CAD build for the part. Positions are in the model's coordinates, mm. Give positions to 0.01 mm unless a question says otherwise; leave off trailing zeros. Order: outer loops, then holes, each group sorted by start corner. A loop starts at its lowest first (then second) coordinate and runs counter-clockwise, first axis right, second up.
Item 1: Flat gauge pins, fed straight in: P1, Ø1, axis at x = 28, y = 3, coming from the +Z side; P2, Ø2, axis at x = 19.5, z = 1, coming from the -Y side. Where does each tip first touch, or does it go through?
Item 2: Band-saw the part on A-A on x = 25. Give the cut face in (y, z).
Item 3: Band-saw the part on B-B on x = 32. Give the cut face in (y, z).
Item 4: Wall check: L1, parallel to X at y = 1.8, z = -1.5 (3 decimals); L2, parallel to Y at x = 32, z = 0.65; L3, parallel to Y at x = 33, z = 0.3. Give the ranges that are in metal, low to high.
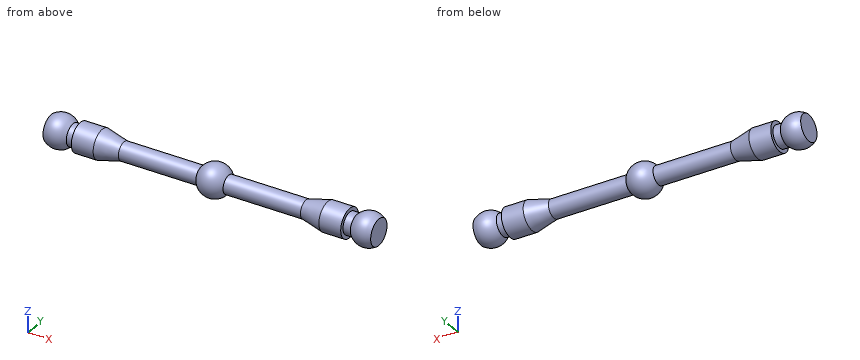
Autodesk Inventor part; units mm, degrees
ref_plane "YZ Plane" through (0, 0, 0) normal (1, 0, 0) x (0, 1, 0)
ref_plane "XZ Plane" through (0, 0, 0) normal (0, 1, 0) x (-1, 0, 0)
ref_plane "XY Plane" through (0, 0, 0) normal (0, 0, 1) x (1, 0, 0)
sketch "Sketch1" plane through (0, 0, 0) normal (0, 0, 1) x (1, 0, 0)
  line L0 (-3.1649, 3.1698) -> (44.3618, 3.1698) construction
  line L1 (4.6175, 4.4198) -> (17.1175, 4.4198) construction
  line L2 (-1.3825, 5.1698) -> (1.6175, 5.1698)
  line L3 (1.6175, 5.1698) -> (4.6175, 4.4198)
  line L4 (17.1175, 14.6605) -> (17.1175, -4.6585) construction
  line L5 (-1.3825, 5.1698) -> (-1.3825, 4.6698)
  line L6 (-1.3825, 4.6698) -> (-2.3825, 4.6698)
  circle A0 centre (-4.0584, 3.1698) radius 2.25 construction
  line L7 (-2.3825, 4.6698) -> (-5.3825, 4.6698) construction
  line L8 (-5.3825, 4.9889) -> (-5.3825, 3.1698)
  arc A1 (-2.3814, 4.6698) -> (-5.3825, 4.9889) centre (-4.0584, 3.1698) ccw
  line L9 (29.6175, 4.4198) -> (17.1175, 4.4198) construction
  line L10 (35.6175, 5.1698) -> (32.6175, 5.1698)
  line L11 (32.6175, 5.1698) -> (29.6175, 4.4198)
  line L12 (35.6175, 5.1698) -> (35.6175, 4.6698)
  line L13 (35.6175, 4.6698) -> (36.6175, 4.6698)
  circle A2 centre (38.2934, 3.1698) radius 2.25 construction
  line L14 (36.6175, 4.6698) -> (39.6175, 4.6698) construction
  line L15 (39.6175, 4.9889) -> (39.6175, 3.1698)
  arc A3 (39.6175, 4.9889) -> (36.6163, 4.6698) centre (38.2934, 3.1698) ccw
  line L16 (-5.3825, 3.1698) -> (39.6175, 3.1698)
  circle A4 centre (17.1175, 3.1698) radius 2.25 construction
  line L17 (4.6175, 4.4198) -> (15.2467, 4.4198)
  arc A5 (18.9883, 4.4198) -> (15.2467, 4.4198) centre (17.1175, 3.1698) ccw
  line L18 (18.9883, 4.4198) -> (29.6175, 4.4198)
  point P0 (37.3999, 3.1698)
  dimension "d1" = 1.25
  dimension "d2" = 12.5
  dimension "d3" = 2
  dimension "d4" = 3
  dimension "d5" = 3
  dimension "d6" = 1.5
  dimension "d7" = 1
  dimension "d8" = 4.5
  dimension "d9" = 3
  dimension "d11" = 4.5
revolve "Revolution1" add sketch "Sketch1" angle 360 about axis through (-5.3825, 3.1698, 0) along (1, 0, 0)
equation "\"d11\" = d8"
properties part number "union"
The answers:
1. P1: stops at z = 1.25
1. P2: stops at y = 1.57
2. outline: circle Ø2.5 at (3.17, 0)
3. outline: circle Ø3.69 at (3.17, 0)
4. L1: x = -5.026 to -3.092, 16.15 to 18.085, 37.327 to 39.261
4. L2: y = 1.44 to 4.9
4. L3: y = 1.19 to 5.15
